from build123d import *

# Parameters (mm, degrees)
BOSS_EXTRUDE1_DEPTH                               = 4.064
CSK_FOR_6_FLAT_HEAD_MACHINE_SCREW_100_D           = 3.7973
CSK_FOR_6_FLAT_HEAD_MACHINE_SCREW_100_CSINK_D     = 7.0866
CSK_FOR_6_FLAT_HEAD_MACHINE_SCREW_100_CSINK_ANGLE = 100
FILLET1_R                                         = 1.016
FILLET2_R                                         = 0.508


with BuildPart() as part:
    # Sketch1 → Boss-Extrude1 (new body, symmetric)
    with BuildSketch(Plane.XY):
        Polygon((0, 0), (0, 1.905), (6.096, 1.905), (6.096, 0), (8.128, 0), (8.128, 3.429), (-8.128, 3.429), (-8.128, 0), align=None)
    extrude(amount=BOSS_EXTRUDE1_DEPTH, both=True)

    # CSK for #6 Flat Head Machine Screw (100)1 (through all)
    with Locations(Plane(origin=(0, 3.429, 0), x_dir=(1, 0, 0), z_dir=(0, 1, 0))):
        with Locations((-4.064, 0)):
            CounterSinkHole(CSK_FOR_6_FLAT_HEAD_MACHINE_SCREW_100_D / 2, CSK_FOR_6_FLAT_HEAD_MACHINE_SCREW_100_CSINK_D / 2, counter_sink_angle=CSK_FOR_6_FLAT_HEAD_MACHINE_SCREW_100_CSINK_ANGLE)

    # Fillet1
    fillet1_edges = [part.edges().sort_by_distance(p)[0] for p in [
        (-8.128, 1.7145, -4.064),
        (8.128, 1.7145, 4.064),
        (8.128, 1.7145, -4.064),
        (-8.128, 1.7145, 4.064),
    ]]
    fillet(fillet1_edges, radius=FILLET1_R)

    # Fillet2
    fillet2_edges = [part.edges().sort_by_distance(p)[0] for p in [
        (8.128, 3.429, 0),
        (0, 3.429, -4.064),
        (-8.128, 3.429, 0),
        (0, 3.429, 4.064),
        (-7.83042049, 3.429, 3.76642049),
        (-7.83042049, 3.429, -3.76642049),
        (7.83042049, 3.429, 3.76642049),
        (7.83042049, 3.429, -3.76642049),
    ]]
    fillet(fillet2_edges, radius=FILLET2_R)


solid = part.part
Read the model definition and answer for the solid it produces. Units are mm, in the model's axes. A direction names the side the tool comes from. Round coordinates to 2 decimals unless told otherwise and drop trailing zeros. Order: outer loops, then holes, each group sorted by start corner. A loop starts at its lowest first (then second) coordinate and runs counter-clockwise, first axis right, second up.
1) The part is cut by section B-B on z = 0. Write down the section's boundary in (x, y) (3 decimals), plus the area to 3 significant figures.
2) The mould has two halves that part along X. Classify faces 3 (the face through (0, 1, 0)), 4 (the face through (-7.838, 1.44, -3.758)), 5 (the face through (8.128, 1, 0)): released by +X, released by -X, zero draft, split by the parting line, or undercut.
3) The part is cut by section C-C on x = 4. Write down the section's boundary in (y, z) (3 decimals), plus the area to 3 significant figures.
4) Flat-ended cylindrical pins translate along their axes: pin 1 (3 mm diameter, centred on x = 6, z = -3, fed in from -Y); pin 2 (3 mm diameter, centred on x = -4.064, z = 0, fed in from -Y). Find the tip coordinate at first contact, or state that the pin passes through.
5) The part is cut by section D-D on y = 2.3. Write down the section's boundary in (x, z), plus the area to 3 significant figures.
6) The part is cut by section A-A on y = 1.35. Write down the section's boundary in (x, z).
7) Straight lines are drawn through the part: L1, parallel to X at y = 0.85, z = 2.75; L2, parallel to Z at x = -3, y = 3.05; L3, parallel to Z at x = -1.25, y = 3.3. For each, find the intervals that lie inside material, in ascending order.
8) For faces 1 (the face through (-2, 1, 4.064)), 2 (the face through (6.096, 1, 0)), determine the directions among +Z, -Z, +X, -X, +Y, -Y from which every point of the face is accessible in a straight line to the end or side of a thin tool.
Resolved:
1. outline: (-8.128, 0) - (-5.963, 0) - (-5.963, 2.049) - (-7.607, 3.429) - (-7.62, 3.429) arc R0.508 ccw to (-8.128, 2.921) - close; (-2.165, 0) - (0, 0) - (0, 1.905) - (6.096, 1.905) - (6.096, 0) - (8.128, 0) - (8.128, 2.921) arc R0.508 ccw to (7.62, 3.429) - (-0.521, 3.429) - (-2.165, 2.049) - close
1. area: 28.7 mm2
2. face 3: undercut
2. face 4: released by -X
2. face 5: released by +X
3. outline: (1.905, -4.064) - (2.921, -4.064) arc R0.508 ccw to (3.429, -3.556) - (3.429, 3.556) arc R0.508 ccw to (2.921, 4.064) - (1.905, 4.064) - close
3. area: 12.3 mm2
4. pin 1: stops at y = 0
4. pin 2: passes through
5. outline: (-8.13, -3.05) arc R1.02 ccw to (-7.11, -4.06) - (7.11, -4.06) arc R1.02 ccw to (8.13, -3.05) - (8.13, 3.05) arc R1.02 ccw to (7.11, 4.06) - (-7.11, 4.06) arc R1.02 ccw to (-8.13, 3.05) - close; hole circle Ø4.4 at (-4.06, 0)
5. area: 116 mm2
6. outline: (-8.13, -3.05) arc R1.02 ccw to (-7.11, -4.06) - (0, -4.06) - (0, 4.06) - (-7.11, 4.06) arc R1.02 ccw to (-8.13, 3.05) - close; (6.1, -4.06) - (7.11, -4.06) arc R1.02 ccw to (8.13, -3.05) - (8.13, 3.05) arc R1.02 ccw to (7.11, 4.06) - (6.1, 4.06) - close; hole circle Ø3.8 at (-4.06, 0)
7. L1: x = -8.13 to 0, 6.1 to 8.13
7. L2: z = -4.05 to -2.9, 2.9 to 4.05
7. L3: z = -3.89 to -1.89, 1.89 to 3.89
8. face 1: +Z, +X, -X, +Y, -Y
8. face 2: +Z, -Z, -Y
